from build123d import *

# Parameters (mm, degrees)
SKETCH1_R                = 1.025
BOSS_EXTRUDE1_DEPTH      = 12
CUT_EXTRUDE1_DEPTH       = 7
BOSS_EXTRUDE2_START      = 4
SKETCH3_R                = 1.025
BOSS_EXTRUDE2_DEPTH      = 4
SKETCH6_R                = 1.025
BOSS_EXTRUDE5_DEPTH      = 7
BOSS_EXTRUDE6_START      = 2
SKETCH7_R                = 1.025
BOSS_EXTRUDE6_DEPTH      = 2
BOSS_EXTRUDE8_DEPTH      = 0.6
BOSS_EXTRUDE8_DEPTH_BACK = 0.6
CUT_EXTRUDE3_START       = -17
SKETCH9_R                = 1.025
CUT_EXTRUDE3_DEPTH       = 17
SKETCH10_R               = 0.9
BOSS_EXTRUDE12_DEPTH     = 14


with BuildPart() as part:
    # Sketch1 → Boss-Extrude1 (new body)
    with BuildSketch(Plane.XY):
        Circle(SKETCH1_R)
    extrude(amount=BOSS_EXTRUDE1_DEPTH)

    # Sketch2 → Cut-Extrude1 (cut)
    with BuildSketch(Plane.XY.offset(12)):
        Polygon((0.866025404, 0), (0.433012702, 0.75), (-0.433012702, 0.75), (-0.866025404, 0), (-0.433012702, -0.75), (0.433012702, -0.75), align=None)
    extrude(amount=-CUT_EXTRUDE1_DEPTH, mode=Mode.SUBTRACT)

    # Sketch3 → Boss-Extrude2 (add)
    with BuildSketch(Plane(origin=(0, 0, 0), x_dir=(-1, 0, 0), z_dir=(0, 0, -1)).offset(BOSS_EXTRUDE2_START)):
        Circle(SKETCH3_R)
    extrude(amount=-BOSS_EXTRUDE2_DEPTH)

    # Sketch6 → Boss-Extrude5 (add)
    with BuildSketch(Plane.XY.offset(12)):
        with Locations(Location((0, 0, 0), (0, 0, 180))):
            Circle(SKETCH6_R)
        Polygon((0.866025404, 0), (0.433012702, 0.75), (-0.433012702, 0.75), (-0.866025404, 0), (-0.433012702, -0.75), (0.433012702, -0.75), align=None, mode=Mode.SUBTRACT)
    extrude(amount=BOSS_EXTRUDE5_DEPTH)

    # Sketch7 → Boss-Extrude6 (add)
    with BuildSketch(Plane(origin=(0, 0, -4), x_dir=(-1, 0, 0), z_dir=(0, 0, -1)).offset(BOSS_EXTRUDE6_START)):
        Circle(SKETCH7_R)
    extrude(amount=-BOSS_EXTRUDE6_DEPTH)

    # Sketch8 → Boss-Extrude8 (add, two sides: drawn at the far end of the back side and taken through both)
    with BuildSketch(Plane(origin=(0, 0, 0), x_dir=(1, 0, 0), z_dir=(0, 1, 0)).offset(-BOSS_EXTRUDE8_DEPTH_BACK)):
        with BuildLine():
            ThreePointArc((0.75, 6), (0, 6.75), (-0.75, 6))
            Line((-0.75, 6), (0.75, 6))
        make_face()
        with BuildLine():
            Line((0.75, 6), (-0.75, 6))
            ThreePointArc((-0.75, 6), (0, 5.25), (0.75, 6))
        make_face()
    extrude(amount=BOSS_EXTRUDE8_DEPTH + BOSS_EXTRUDE8_DEPTH_BACK)

    # Sketch9 → Cut-Extrude3 (cut)
    with BuildSketch(Plane.XY.offset(19).offset(CUT_EXTRUDE3_START)):
        with Locations(Location((0, 0, 0), (0, 0, 180))):
            Circle(SKETCH9_R)
    extrude(amount=CUT_EXTRUDE3_DEPTH, mode=Mode.SUBTRACT)

    # Sketch10 → Boss-Extrude12 (add)
    with BuildSketch(Plane.XY.offset(2)):
        Circle(SKETCH10_R)
        Polygon((0.75055535, 0), (0.375277675, 0.65), (-0.375277675, 0.65), (-0.75055535, 0), (-0.375277675, -0.65), (0.375277675, -0.65), align=None, mode=Mode.SUBTRACT)
    extrude(amount=BOSS_EXTRUDE12_DEPTH)


solid = part.part
For this review, take the finished solid that the model builds, in its own axes (mm). A direction names the side the tool comes from. Round coordinates to 2 decimals unless told otherwise and drop trailing zeros. Write each loop counter-clockwise with the first axis right and the second up, starting at its lowest first coordinate (ties: lowest second). Pieces come first, ordered by that corner, then holes. Notation, with made-up numbers: (-18.75, 27) - (-0.75, 27) arc R19 cw to (-0.75, 31) - close; hole circle Ø5 at (-38, 15.25). An arc over 180 degrees is marked (long way). Use a Markdown table: item, result.
Q1. We need section C-C (y = -0.3). Give the boundary of the cut face in (x, z), plus the area to 3 significant figures.
Derived:
| item | result |
|---|---|
| outline | (-0.98, -6) - (-0.75, -6) arc R0.75 ccw to (0.75, -6) - (0.98, -6) - (0.98, 2) - (0.85, 2) - (0.85, 16) - (0.58, 16) - (0.58, 2) - (-0.58, 2) - (-0.58, 16) - (-0.85, 16) - (-0.85, 2) - (-0.98, 2) - close |
| area | 24.2 mm2 |
Q2. Wall thickness on line 1 along X through (y, z) = (0.05, 1.5); line 2 along Z through (x, y) = (-0.1, -0.7); line 3 along Z through (x, y) = (0.05, -0.35): over which ranges is each line inside the solid? List them lowest first.
Derived:
| item | result |
|---|---|
| line 1 | x = -1.02 to 1.02 |
| line 2 | z = -6 to 16 |
| line 3 | z = -6.75 to 2 |
Q3. Clearance check with flat-ended pins moving along their axes: pin 1 (0.6 mm diameter, centred on x = 0, z = -6.5, fed in from +Y); pin 2 (0.6 mm diameter, centred on x = 0, y = 0, fed in from +Z). State where each tip first meets the part, or that it passes through.
Derived:
| item | result |
|---|---|
| pin 1 | stops at y = 0.6 |
| pin 2 | stops at z = 2 |
Q4. We need section A-A (z = 10.25). Give the boundary of the cut face in (x, y).
Derived:
| item | result |
|---|---|
| outline | circle Ø1.8 at (0, 0); hole (-0.75, 0) - (-0.38, -0.65) - (0.38, -0.65) - (0.75, 0) - (0.38, 0.65) - (-0.38, 0.65) - close |
Q5. We need section B-B (x = 0). Give the boundary of the cut face in (y, z) (3 decimals), plus the area to 3 significant figures.
Derived:
| item | result |
|---|---|
| outline | (-1.025, -6) - (-0.6, -6) - (-0.6, -6.75) - (0.6, -6.75) - (0.6, -6) - (1.025, -6) - (1.025, 2) - (0.9, 2) - (0.9, 16) - (0.65, 16) - (0.65, 2) - (-0.65, 2) - (-0.65, 16) - (-0.9, 16) - (-0.9, 2) - (-1.025, 2) - close |
| area | 24.3 mm2 |
Q6. Machinability: for faces 3 (the cylindrical face through (0.86, 0.27, 8.9)), 4 (the cylindrical face through (0.02, -0.01, -6.75)), which of the approach directions +Z, -Z, +X, -X, +Y, -Y give a long, thin tool a straight path to every point of the face, cutting with its end or side? Answer none if there is none.
Derived:
| item | result |
|---|---|
| face 3 | +Z |
| face 4 | -Z, +Y, -Y |
Q7. We need section D-D (z = -5.25). Give the boundary of the cut face in (x, y) (3 decimals), plus the area to 3 significant figures.
Derived:
| item | result |
|---|---|
| outline | circle Ø2.05 at (0, 0) |
| area | 3.30 mm2 |
Q8. The part is to be moulded in two halves that separate along X. For faces 1 (the cylindrical face through (-0.068, 1.023, -2.056)), 2 (the flat face through (0, 0, 2)), say which applies: pulls with the +X half, pulls with the -X half, needs draft (parallel to the pull), parting line crosses it, or undercut.
Derived:
| item | result |
|---|---|
| face 1 | parting line crosses it |
| face 2 | undercut |
